The figure shows three views and two pictorial views of one solid part (mm, origin at its lowest corner). Answer the questions. A direction names the side the tool comes from. Round coordinates to 2 decimals unless told otherwise and drop trailing zeros. Order: outer loops, then holes, each group sorted by start corner. A loop starts at its lowest first (then second) coordinate and runs counter-clockwise, first axis right, second up. Notation, with made-up numbers: (73.25, 14) -> (88.25, 14) arc R26 cw to (88.25, 48) -> close; hole circle Ø10 at (-35, 87). An arc over 180 degrees is marked (long way). Return JSON: item names as keys, results as strings. Group by question number.
(1) Which of the six approach directions +Z, -Z, +X, -X, +Y, -Y give full straight-line access (tool end or side, diameter ignored) to the marked faces 1, 2 and 3?
(2) The part is cut by section B-B (z = 3.3). Determine the outline of the cut face in (x, y), plus the area to 3 significant figures.
(3) The part is cut by section A-A (x = 3.9). Determine the outline of the cut face in (y, z), plus the area to 3 significant figures.
(4) The part is cut by section C-C (y = 0.8). Determine the outline of the cut face in (x, z), plus the area to 3 significant figures.
(5) Each of these flat-tipped pins is pushed along its axis until it touches: pin 1 (2 mm diameter, centred on y = 3, z = 3.5, fed in from -X); pin 2 (0.5 mm diameter, centred on x = 4, z = 8.5, fed in from +Y). Where does it stop, or does it pass through?
(6) Consider line 1 (Y direction, x = 1.75, z = 7.25); line 2 (Y direction, x = 2.5, z = 8.5); line 3 (Z direction, x = 4, y = 1.85). Determine where each line is inside the solid, lowest interval first. Write a range as [from, to].
(7) The part is cut by section D-D (x = 2.5). Determine the outline of the cut face in (y, z), plus the area to 3 significant figures.
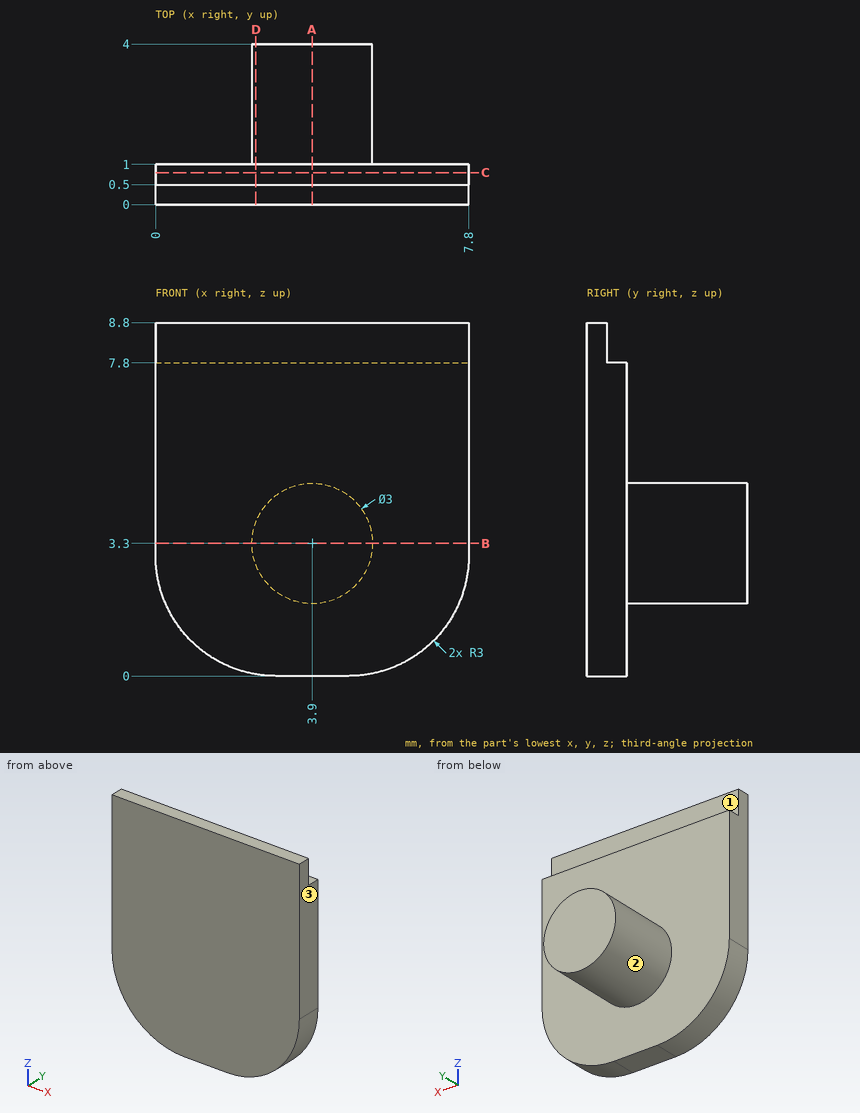
Answer below:
{
 "1": {"face 1": "+Z, +X, -X, +Y", "face 2": "+Y", "face 3": "+Z, -Z, +X, +Y, -Y"},
 "2": {"outline": "(0, 0) -> (7.8, 0) -> (7.8, 1) -> (5.4, 1) -> (5.4, 4) -> (2.4, 4) -> (2.4, 1) -> (0, 1) -> close", "area": "16.8 mm²"},
 "3": {"outline": "(0, 0) -> (1, 0) -> (1, 1.8) -> (4, 1.8) -> (4, 4.8) -> (1, 4.8) -> (1, 7.8) -> (0.5, 7.8) -> (0.5, 8.8) -> (0, 8.8) -> close", "area": "17.3 mm²"},
 "4": {"outline": "(0, 3) arc R3 ccw to (3, 0) -> (4.8, 0) arc R3 ccw to (7.8, 3) -> (7.8, 7.8) -> (0, 7.8) -> close", "area": "57.0 mm²"},
 "5": {"pin 1": "stops at x = 2.4", "pin 2": "stops at y = 0.5"},
 "6": {"line 1": "y = [0, 1]", "line 2": "y = [0, 0.5]", "line 3": "z = [1.8, 4.8]"},
 "7": {"outline": "(0, 0.04) -> (1, 0.04) -> (1, 2.76) -> (4, 2.76) -> (4, 3.84) -> (1, 3.84) -> (1, 7.8) -> (0.5, 7.8) -> (0.5, 8.8) -> (0, 8.8) -> close", "area": "11.5 mm²"}
}
